Here's how the part is built. I have some questions about the finished solid (model axes, mm). Face numbers are marked on the shaded views. A direction names the side the tool comes from. Give positions to 0.01 mm unless a question says otherwise; leave off trailing zeros. Loops run counter-clockwise (first coordinate to the right, second up) from the corner with the lowest first, then second, coordinate; pieces in that order, holes last. Notation, with made-up numbers: M 8,-8 L 55,-8 A13 cw 55,4 Z; hole C 11.25,8.5 d3. An arc over 180 degrees is marked long. Answer as CSV lines item,"result". Start each with the question number.
Item 1: If I drill on line 1 along X through (y, z) = (7.5, -46) (3 decimals); line 2 along X through (y, z) = (-6, 55.5); line 3 along Z through (x, y) = (26, -5.5), over which ranges is the centre line in solid material (lowest first)? Write a range as from..to.
Item 2: For the marked faces 1, 2 and 3, which set-ups out of +Z, -Z, +X, -X, +Y, -Y let a thin tool reach every point of the face, with its end or its side?
Item 3: I want a section at A-A on x = 23. List the corners of the cut face in (y, z) for me (3 decimals), plus the area to 3 significant figures.
Item 4: I want a section at D-D on x = -8. List the corners of the cut face in (y, z) for me (3 decimals), plus the area to 3 significant figures.
Item 5: I want a section at B-B on z = -34. List the corners of the cut face in (x, y) for me (3 decimals), plus the area to 3 significant figures.
Item 6: I want a section at C-C on y = 4.5. List the corners of the cut face in (x, z) for me (3 decimals), plus the area to 3 significant figures.
Item 7: If we mould it in two halves opening along X, with no side actions, what happens to the marked faces 4, 5 and 6? For each: released by +X, released by -X, zero draft, split by the parting line, or undercut.
Item 8: Will these pins go through, and if not, where does the flat tip stop? P1, Ø1.5, axis at x = -4.5, y = 0, coming from the -Z side; P2, Ø1, axis at x = 33.5, z = 34, coming from the +Y side; P3, Ø8, axis at y = 22.5, z = -28, coming from the +X side (3 decimals); P4, Ø8, axis at x = 24, y = 7.5, coming from the +Z side.
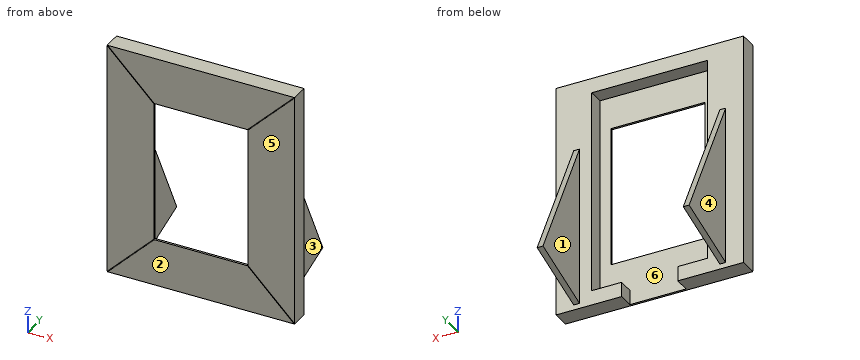
from build123d import *

# Parameters (mm, degrees)
F2_W              = 101.854
F2_H              = 127.3048
F2_W_2            = 51.054
F2_H_2            = 76.5048
F3_DEPTH          = 9.525
F4_W              = 62.992
F4_H              = 111.252
F5_DEPTH          = 8.382
F8_DEPTH          = 3.175
F9_W              = 30.48
F9_H              = 8.0264
F10_DEPTH         = 8.382
F12_DEPTH         = 0.254
F12_COPIES2_COUNT = 2


# Not quite as in the source:
# - a pattern or mirror of a feature is missing from the dataset's text; its kind, count and spacing are read off the source's solid


with BuildPart() as f3:
    # F2 (on Front) → F3 (new body)
    with BuildSketch(Plane.XZ):
        Rectangle(F2_W, F2_H)
        Rectangle(F2_W_2, F2_H_2, mode=Mode.SUBTRACT)
    extrude(amount=F3_DEPTH)

    # F4 (on face) → F5 (cut)
    with BuildSketch(Plane(origin=(0, 0, 0), x_dir=(-1, 0, 0), z_dir=(0, 1, 0))):
        Rectangle(F4_W, F4_H)
    extrude(amount=-F5_DEPTH, mode=Mode.SUBTRACT)

    # F7 (on offset) → F8 (join)
    with BuildSketch(Plane.YZ.offset(38.1)):
        Polygon((37.1396206319, -48.7135574222), (0, 25.9003154933), (0, -60.8499720693), align=None)
    f8 = extrude(amount=F8_DEPTH)

    # F8_copies: F8 across plane
    add(f8.mirror(Plane(origin=(0, 0, 0), x_dir=(0, 0, -1), z_dir=(-1, 0, 0))))

    # F9 (on face) → F10 (cut, through all)
    with BuildSketch(Plane(origin=(0, 0, 0), x_dir=(-1, 0, 0), z_dir=(0, 1, 0))):
        with Locations((0, -59.6392)):
            Rectangle(F9_W, F9_H)
    extrude(amount=-F10_DEPTH, mode=Mode.SUBTRACT)

    # F11 (on face) → F12 (cut)
    with BuildSketch(Plane.XZ.offset(9.525)):
        Polygon((-50.927, 63.3984), (-25.527, 37.9984), (-25.527, 38.2524), (-25.273, 38.2524), (-50.673, 63.6524), (-50.927, 63.6524), align=None)
    f12 = extrude(amount=-F12_DEPTH, mode=Mode.SUBTRACT)

    # F12_copies: F12 across plane
    add(f12.mirror(Plane(origin=(0, 0, 0), x_dir=(0, 0, 1), z_dir=(1, 0, 0))), mode=Mode.SUBTRACT)

    # F12_copies1: F12 across plane
    add(f12.mirror(Plane(origin=(0, 0, 0), x_dir=(-1, 0, 0), z_dir=(0, 0, -1))), mode=Mode.SUBTRACT)

    # F12_copies2: F12 ×2 about axis
    f12_copies2_axis = Axis((0, 0, 0), (0, 1, 0))
    for i in range(1, F12_COPIES2_COUNT):
        add(f12.rotate(f12_copies2_axis, i * 360 / F12_COPIES2_COUNT), mode=Mode.SUBTRACT)


solid = f3.part
Result:
1,line 1,"-41.275..-38.1, 38.1..41.275"
1,line 2,"-50.93..-31.5, 31.5..50.93"
1,line 3,"-63.65..-55.63, 55.63..63.65"
2,face 1,"+Z, -Z, +Y"
2,face 2,"+Z, -Z, +X, -X, -Y"
2,face 3,"+Z, -Z, +X, +Y"
3,outline,"M -9.525,-63.652 L 0,-63.652 L 0,-55.626 L -8.382,-55.626 L -8.382,-38.252 L -9.525,-38.252 Z; M -9.525,38.252 L -8.382,38.252 L -8.382,55.626 L 0,55.626 L 0,63.652 L -9.525,63.652 Z"
3,area,"193 mm^2"
4,outline,"M -9.525,-63.652 L -8.382,-63.652 L -8.382,-38.252 L -9.525,-38.252 Z; M -9.525,38.252 L -8.382,38.252 L -8.382,55.626 L 0,55.626 L 0,63.652 L -9.525,63.652 Z"
4,area,"125 mm^2"
5,outline,"M -50.927,-9.525 L -25.527,-9.525 L -25.527,-8.382 L -31.496,-8.382 L -31.496,0 L -38.1,0 L -38.1,29.816 L -41.275,29.816 L -41.275,0 L -50.927,0 Z; M 25.527,-9.525 L 50.927,-9.525 L 50.927,0 L 41.275,0 L 41.275,29.816 L 38.1,29.816 L 38.1,0 L 31.496,0 L 31.496,-8.382 L 25.527,-8.382 Z"
5,area,"573 mm^2"
6,outline,"M -41.275,-59.379 L -38.1,-59.379 L -38.1,16.86 L -41.275,16.86 Z; M 38.1,-59.379 L 41.275,-59.379 L 41.275,16.86 L 38.1,16.86 Z"
6,area,"484 mm^2"
7,face 4,"released by -X"
7,face 5,"zero draft"
7,face 6,"undercut"
8,P1,"z = 55.63"
8,P2,"y = 0"
8,P3,"x = 41.275"
8,P4,"through"
